Read the model definition and answer for the solid it produces. Units are mm, in the model's axes. Face numbers are marked on the shaded views. A direction names the side the tool comes from. Coordinates: 2 decimals unless noted, no trailing zeros. Write each loop counter-clockwise with the first axis right and the second up, starting at its lowest first coordinate (ties: lowest second). Pieces come first, ordered by that corner, then holes. Notation, with made-up numbers: (-24.75, 17) - (0.25, 17) arc R12 cw to (0.25, 36) - close; hole circle Ø8 at (42, -1.5). An arc over 180 degrees is marked (long way). Use a Markdown table: item, result.
from build123d import *

# Parameters (mm, degrees)
F0_W     = 99.0809351206
F0_H     = 58.4763474762
F0_R     = 16.3683146095
F1_DEPTH = 12.7
F2_R     = 21.8636685636
F3_DEPTH = 25.4
F4_R     = 5.08
F5_R     = 14.8918944932
F6_DEPTH = 3.175
F7_R     = 21.1028142618
F7_R_2   = 14.8918944932
F8_DEPTH = 25.4
F9_R     = 5.08
F11_D    = 6.35
F12_R    = 5.08


with BuildPart() as f1:
    # F0 (on Top) → F1 (new body)
    with BuildSketch(Plane.XY):
        Rectangle(F0_W, F0_H)
        Circle(F0_R, mode=Mode.SUBTRACT)
        Circle(F0_R)
    extrude(amount=F1_DEPTH)

    # F2 (on face) → F3 (join)
    with BuildSketch(Plane.XY.offset(12.7)):
        Circle(F2_R)
    extrude(amount=F3_DEPTH)

    # F4
    f4_edges = [f1.edges().sort_by_distance(p)[0] for p in [
        (0, 29.238174, 12.7),
        (49.540468, 0, 12.7),
        (0, -29.238174, 12.7),
        (-49.540468, 0, 12.7),
    ]]
    fillet(f4_edges, radius=F4_R)

    # F5 (on face) → F6 (join)
    with BuildSketch(Plane.XY.offset(38.1)):
        Circle(F5_R)
    extrude(amount=F6_DEPTH)

    # F7 (on face) → F8 (join)
    with BuildSketch(Plane.XY.offset(41.275)):
        Circle(F7_R)
        Circle(F7_R_2, mode=Mode.SUBTRACT)
        Circle(F7_R_2)
    extrude(amount=F8_DEPTH)

    # F9
    f9_edges = [f1.edges().sort_by_distance(p)[0] for p in [
        (-21.102814, 0, 41.275),
        (-21.863669, 0, 38.1),
    ]]
    fillet(f9_edges, radius=F9_R)

    # F11 (through all)
    with Locations(Plane.XY.offset(12.7)):
        with Locations((38.6345759034, 17.8116075695), (38.0743406713, -18.4829942882), (-36.1839905381, 16.3736771792), (-38.3434481919, -18.9137440175)):
            Hole(F11_D / 2)

    # F12
    f12_edges = [f1.edges().sort_by_distance(p)[0] for p in [
        (-21.102814, 0, 66.675),
    ]]
    fillet(f12_edges, radius=F12_R)


solid = f1.part
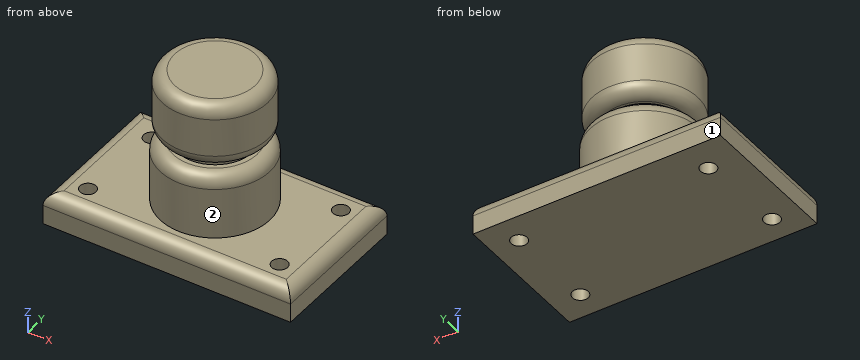
(1) A cutting plane is placed at B-B, the plane y = 0. Write down the section's boundary in (x, z) (3 decimals).
Report:
| item | result |
|---|---|
| outline | (-49.54, 0) - (49.54, 0) - (49.54, 7.62) arc R5.08 ccw to (44.46, 12.7) - (21.864, 12.7) - (21.864, 33.02) arc R5.08 ccw to (16.784, 38.1) - (14.892, 38.1) - (14.892, 41.275) - (16.023, 41.275) arc R5.08 ccw to (21.103, 46.355) - (21.103, 61.595) arc R5.08 ccw to (16.023, 66.675) - (-16.023, 66.675) arc R5.08 ccw to (-21.103, 61.595) - (-21.103, 46.355) arc R5.08 ccw to (-16.023, 41.275) - (-14.892, 41.275) - (-14.892, 38.1) - (-16.784, 38.1) arc R5.08 ccw to (-21.864, 33.02) - (-21.864, 12.7) - (-44.46, 12.7) arc R5.08 ccw to (-49.54, 7.62) - close |
(2) A cutting plane is placed at A-A, the plane x = 0. Write down the section's boundary in (y, z) (3 decimals), and give its area (3 significant figures).
Report:
| item | result |
|---|---|
| outline | (-29.238, 0) - (29.238, 0) - (29.238, 7.62) arc R5.08 ccw to (24.158, 12.7) - (21.864, 12.7) - (21.864, 33.02) arc R5.08 ccw to (16.784, 38.1) - (14.892, 38.1) - (14.892, 41.275) - (16.023, 41.275) arc R5.08 ccw to (21.103, 46.355) - (21.103, 61.595) arc R5.08 ccw to (16.023, 66.675) - (-16.023, 66.675) arc R5.08 ccw to (-21.103, 61.595) - (-21.103, 46.355) arc R5.08 ccw to (-16.023, 41.275) - (-14.892, 41.275) - (-14.892, 38.1) - (-16.784, 38.1) arc R5.08 ccw to (-21.864, 33.02) - (-21.864, 12.7) - (-24.158, 12.7) arc R5.08 ccw to (-29.238, 7.62) - close |
| area | 2,980 mm² |
(3) Straight lines are drawn through the part: L1, parallel to Y at x = 41, z = 3; L2, parallel to X at y = -14, z = 28; L3, parallel to Z at x = -24.5, y = 23.5. For each, find the intervals that lie inside material, in ascending order.
Report:
| item | result |
|---|---|
| L1 | y = -29.24 to -19.72, -17.25 to 15.69, 19.93 to 29.24 |
| L2 | x = -16.79 to 16.79 |
| L3 | z = 0 to 12.7 |
(4) A cutting plane is placed at D-D, the plane z = 39.5. Write down the section's boundary in (x, y).
Report:
| item | result |
|---|---|
| outline | circle Ø29.78 at (0, 0) |
(5) A cutting plane is placed at C-C, the plane z = 5.5. Write down the section's boundary in (x, y) (3 decimals).
Report:
| item | result |
|---|---|
| outline | (-49.54, -29.238) - (49.54, -29.238) - (49.54, 29.238) - (-49.54, 29.238) - close; hole circle Ø6.35 at (-38.343, -18.914); hole circle Ø6.35 at (-36.184, 16.374); hole circle Ø6.35 at (38.074, -18.483); hole circle Ø6.35 at (38.635, 17.812) |
(6) Each of these flat-tipped pins is pushed along its axis until it touches: P1, Ø3, axis at x = 3.5, z = 9.5, coming from the +Y side; P2, Ø1, axis at x = -0.5, z = 41.5, coming from the -Y side; P3, Ø8.5, axis at x = -38.34, y = -18.91, coming from the +Z side; P4, Ø4, axis at x = 38.63, y = 17.81, coming from the +Z side. Where does it stop, or does it pass through?
Report:
| item | result |
|---|---|
| P1 | stops at y = 29.22 |
| P2 | stops at y = -18.63 |
| P3 | stops at z = 12.7 |
| P4 | passes through |
(7) For the marked faces 1 and 2, determine the directions among +Z, -Z, +X, -X, +Y, -Y from which every point of the face is accessible in a straight line to the end or side of a thin tool.
Report:
| item | result |
|---|---|
| face 1 | +Z, -Z, +X, -X, +Y |
| face 2 | +Z |
